Design review of the part built by this model. Coordinates are the model's own, in mm. Face numbers are marked on the shaded views. Round coordinates to 2 decimals unless told otherwise and drop trailing zeros. Write each loop counter-clockwise with the first axis right and the second up, starting at its lowest first coordinate (ties: lowest second). Pieces come first, ordered by that corner, then holes.
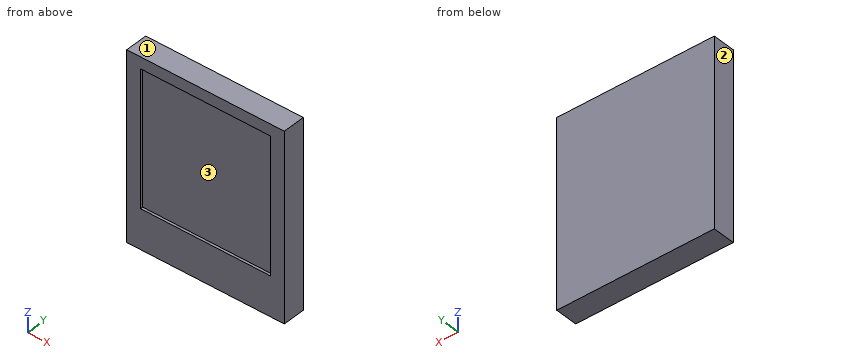
from build123d import *

# Parameters (mm, degrees)
F0_W     = 30.9
F0_H     = 36.51
F1_DEPTH = 4.4
F2_W     = 25.4976
F2_H     = 26.496
F3_DEPTH = 0.5


with BuildPart() as f1:
    # F0 (on Front) → F1 (new body)
    with BuildSketch(Plane.XZ):
        with Locations((0, -2.747)):
            Rectangle(F0_W, F0_H)
    extrude(amount=F1_DEPTH)

    # F2 (on face) → F3 (cut)
    with BuildSketch(Plane.XZ.offset(4.4)):
        Rectangle(F2_W, F2_H)
    extrude(amount=-F3_DEPTH, mode=Mode.SUBTRACT)


solid = f1.part
1) For P1, Ø10, axis at x = 0, z = 2, coming from the -Y side, flat-tipped, find the tip position at first contact; note if it passes through.
2) Add section A-A on x = 6. State the section outline as (y, z) points.
3) Add section B-B on z = -10. State the section outline as (x, y) points.
4) The part is to be moulded in two halves that separate along Z. For the marked faces 1, 2 and 3, say which applies: pulls with the +Z half, pulls with the -Z half, needs draft (parallel to the pull), parting line crosses it, or undercut.
5) For line 1 along Z through (x, y) = (7, -4); line 2 along Y through (x, z) = (-10, 5), list the stretches that pass through material, from the lowest coordinate up.
Computed:
1. P1: stops at y = -3.9
2. outline: (-4.4, -21) - (0, -21) - (0, 15.51) - (-4.4, 15.51) - (-4.4, 13.25) - (-3.9, 13.25) - (-3.9, -13.25) - (-4.4, -13.25) - close
3. outline: (-15.45, -4.4) - (-12.75, -4.4) - (-12.75, -3.9) - (12.75, -3.9) - (12.75, -4.4) - (15.45, -4.4) - (15.45, 0) - (-15.45, 0) - close
4. face 1: pulls with the +Z half
4. face 2: needs draft
4. face 3: undercut
5. line 1: z = -21 to -13.25, 13.25 to 15.51
5. line 2: y = -3.9 to 0
